Can you work these out from the drawing? Everything is in mm from the part's minimum corner. Coordinates: 2 decimals unless noted, no trailing zeros. Order: outer loops, then holes, each group sorted by start corner. A loop starts at its lowest first (then second) coordinate and runs counter-clockwise, first axis right, second up. Notation, with made-up numbers: (-7.75, 59.5) -> (4.25, 59.5) arc R22 ccw to (4.25, 87.5) -> close; hole circle Ø4 at (83, -16.75). An arc over 180 degrees is marked (long way). Return JSON: item names as keys, results as strings. Group by question number.
1) If we section it at D-D, the plane x = 44.45: Please give me the cut outline in (y, z) (1 decimal).
2) If we section it at C-C, the plane y = 0.85: State how many separate pieces and enclosed holes the cut face has, then the cut area to 3 significant figures.
3) For pin 1 (5.5 mm diameter, centred on x = 95.25, z = 108.74, fed in from +Y), with a flat end and sliding along its axis, tell me the tip position at first contact or that it passes through.
4) If I drill on probe 1 along Z at (x, y) = (146.05, 0.95) (1 decimal); probe 2 along X at (y, z) = (1.35, 73); probe 3 along X at (y, z) = (1.95, 8) (1 decimal), over which ranges is the centre line in solid material (lowest first)? Write a range as from..to.
5) If we section it at A-A, the plane x = 171.45: Please give me the cut outline in (y, z).
6) If we section it at B-B, the plane z = 96.5: Please give me the cut outline in (x, y), then the cut area to 3 significant figures.
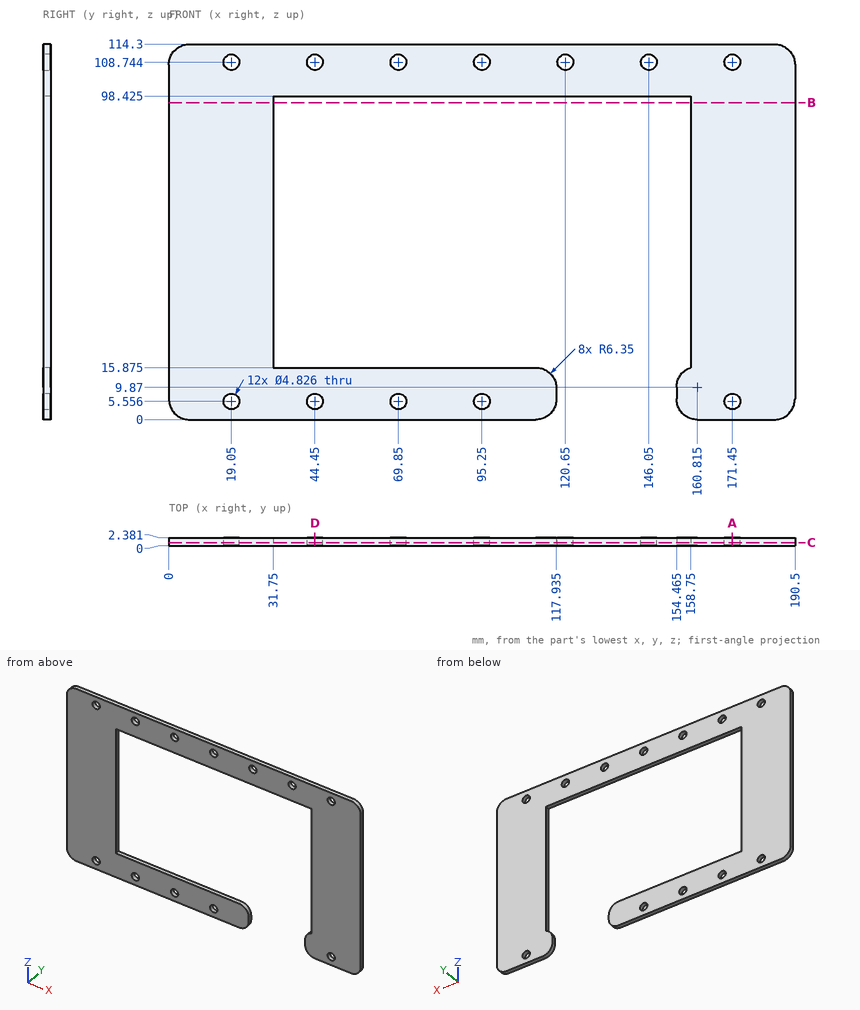
Result sheet:
{
 "1": {"outline": "(0, 0) -> (2.4, 0) -> (2.4, 3.1) -> (0, 3.1) -> close; (0, 8) -> (2.4, 8) -> (2.4, 15.9) -> (0, 15.9) -> close; (0, 98.4) -> (2.4, 98.4) -> (2.4, 106.3) -> (0, 106.3) -> close; (0, 111.2) -> (2.4, 111.2) -> (2.4, 114.3) -> (0, 114.3) -> close"},
 "2": {"separate pieces": "1", "enclosed holes": "12", "area": "10,400 mm2"},
 "3": {"pin 1": "stops at y = 2.38"},
 "4": {"probe 1": "z = 98.4..106.3, 111.2..114.3", "probe 2": "x = 0..31.75, 158.75..190.5", "probe 3": "x = 0..117.9, 154.5..190.5"},
 "5": {"outline": "(0, 0) -> (2.38, 0) -> (2.38, 3.14) -> (0, 3.14) -> close; (0, 7.97) -> (2.38, 7.97) -> (2.38, 106.33) -> (0, 106.33) -> close; (0, 111.16) -> (2.38, 111.16) -> (2.38, 114.3) -> (0, 114.3) -> close"},
 "6": {"outline": "(0, 0) -> (31.75, 0) -> (31.75, 2.38) -> (0, 2.38) -> close; (158.75, 0) -> (190.5, 0) -> (190.5, 2.38) -> (158.75, 2.38) -> close", "area": "151 mm2"}
}
